Read the model definition and answer for the solid it produces. Units are mm, in the model's axes. Face numbers are marked on the shaded views. A direction names the side the tool comes from. Give positions to 0.01 mm unless a question says otherwise; leave off trailing zeros. Loops run counter-clockwise (first coordinate to the right, second up) from the corner with the lowest first, then second, coordinate; pieces in that order, holes last.
(1) Determine the mould class of the marked faces 3, 4, 5 and 6 for opening direction Y: pulls with the +Y half, pulls with the -Y half, needs draft (parallel to the pull), parting line crosses it, or undercut.
(2) Find section A-A, the plane y = 56. Write down the section's boundary in (x, z), then the cut area to 3 significant figures.
(3) Find section B-B, the plane x = 81.5. Write down the section's boundary in (y, z), then the cut area to 3 significant figures.
(4) Which of the six approach directions +Z, -Z, +X, -X, +Y, -Y give full straight-line access (tool end or side, diameter ignored) to the marked faces 1 and 2?
(5) Find section C-C, the plane z = -22.5. Write down the section's boundary in (x, y).
(6) Straight lines are drawn through the part: probe 1 along Y at (x, z) = (65, -12); probe 2 along Y at (x, z) = (72.5, 32); probe 3 along X at (y, z) = (49.5, 47). For each, find the intervals that lie inside material, in ascending order.
(7) This flat-tipped pin is pushed along its axis until it touches: P1, Ø16, axis at x = 75.21, y = 75.82, coming from the +Z side. Where does it stop, or does it pass through?
(8) Find section D-D, the plane y = 82. Write down the section's boundary in (x, z).
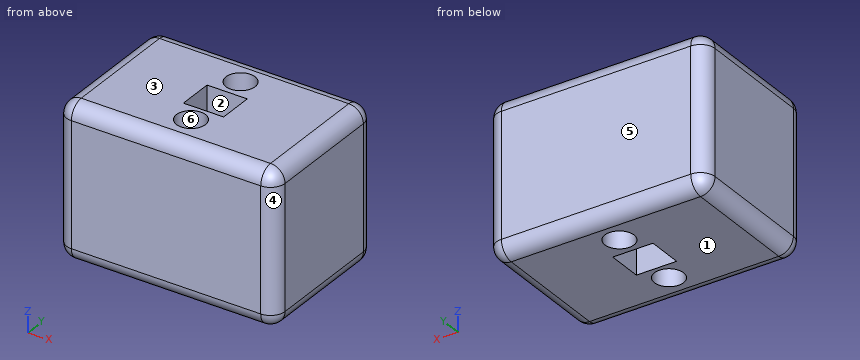
```python
from build123d import *

# Parameters (mm, degrees)
SKETCH1_W                = 150
SKETCH1_H                = 100
BOSS_EXTRUDE1_DEPTH      = 60
BOSS_EXTRUDE1_DEPTH_BACK = 45
SKETCH5_W                = 27.629917719
SKETCH5_H                = 24.20295118
CUT_EXTRUDE1_DEPTH       = 79
CUT_EXTRUDE1_DEPTH_BACK  = 83
FILLET1_R                = 10
SKETCH7_R                = 10
CUT_EXTRUDE2_DEPTH       = 125


with BuildPart() as part:
    # Sketch1 → Boss-Extrude1 (new body, two sides)
    with BuildSketch(Plane.XY) as boss_extrude1_sk:
        with Locations((75, 50)):
            Rectangle(SKETCH1_W, SKETCH1_H)
    extrude(amount=BOSS_EXTRUDE1_DEPTH)
    extrude(boss_extrude1_sk.sketch, amount=-BOSS_EXTRUDE1_DEPTH_BACK)

    # Sketch5 → Cut-Extrude1 (cut, two sides)
    with BuildSketch(Plane(origin=(42.452521569, 36, 0), x_dir=(1, 0, 0), z_dir=(0, 0, 1))) as cut_extrude1_sk:
        with Locations((32.75337542, 14.030268891)):
            Rectangle(SKETCH5_W, SKETCH5_H)
    extrude(amount=CUT_EXTRUDE1_DEPTH, mode=Mode.SUBTRACT)
    extrude(cut_extrude1_sk.sketch, amount=-CUT_EXTRUDE1_DEPTH_BACK, mode=Mode.SUBTRACT)

    # Fillet1
    fillet1_edges = [part.edges().sort_by_distance(p)[0] for p in [
        (75, 0, -45),
        (0, 50, -45),
        (75, 100, -45),
        (150, 50, -45),
        (75, 100, 60),
        (0, 50, 60),
        (75, 0, 60),
        (0, 0, 7.5),
        (0, 100, 7.5),
        (150, 100, 7.5),
        (150, 0, 7.5),
        (150, 50, 60),
    ]]
    fillet(fillet1_edges, radius=FILLET1_R)

    # Sketch7 → Cut-Extrude2 (cut, symmetric)
    with BuildSketch(Plane.XY):
        with Locations((75.20589699, 75.819077446)):
            Circle(SKETCH7_R)
        with Locations((75.20589699, 25.173963995)):
            Circle(SKETCH7_R)
    extrude(amount=CUT_EXTRUDE2_DEPTH, both=True, mode=Mode.SUBTRACT)


solid = part.part
```
Entries:
1. face 3: needs draft
1. face 4: pulls with the -Y half
1. face 5: pulls with the +Y half
1. face 6: undercut
2. outline: (0, -35) arc R10 ccw to (10, -45) - (61.39, -45) - (61.39, 60) - (10, 60) arc R10 ccw to (0, 50) - close; (89.02, -45) - (140, -45) arc R10 ccw to (150, -35) - (150, 50) arc R10 ccw to (140, 60) - (89.02, 60) - close
2. area: 12,800 mm2
3. outline: (0, -35) arc R10 ccw to (10, -45) - (17.4, -45) - (17.4, 60) - (10, 60) arc R10 ccw to (0, 50) - close; (32.94, -45) - (37.93, -45) - (37.93, 60) - (32.94, 60) - close; (62.13, -45) - (68.05, -45) - (68.05, 60) - (62.13, 60) - close; (83.59, -45) - (90, -45) arc R10 ccw to (100, -35) - (100, 50) arc R10 ccw to (90, 60) - (83.59, 60) - close
3. area: 4,610 mm2
4. face 1: -Z, +X, -X, +Y, -Y
4. face 2: +Z, -Z
5. outline: (0, 10) arc R10 ccw to (10, 0) - (140, 0) arc R10 ccw to (150, 10) - (150, 90) arc R10 ccw to (140, 100) - (10, 100) arc R10 ccw to (0, 90) - close; hole (61.39, 37.93) - (89.02, 37.93) - (89.02, 62.13) - (61.39, 62.13) - close; hole circle Ø20 at (75.21, 25.17); hole circle Ø20 at (75.21, 75.82)
6. probe 1: y = 0 to 37.93, 62.13 to 100
6. probe 2: y = 0 to 15.55, 34.8 to 37.93, 62.13 to 66.19, 85.45 to 100
6. probe 3: x = 0 to 61.39, 89.02 to 150
7. P1: passes through
8. outline: (0, -35) arc R10 ccw to (10, -45) - (67.34, -45) - (67.34, 60) - (10, 60) arc R10 ccw to (0, 50) - close; (83.07, -45) - (140, -45) arc R10 ccw to (150, -35) - (150, 50) arc R10 ccw to (140, 60) - (83.07, 60) - close
